from build123d import *

# Parameters (mm, degrees)
SKETCH1_W           = 63.5
SKETCH1_H           = 21.59
BOSS_EXTRUDE1_DEPTH = 5.08
SKETCH2_W           = 19.05
SKETCH2_H           = 20.32
BOSS_EXTRUDE2_DEPTH = 1.27
SKETCH3_W           = 1.27
SKETCH3_H           = 21.59
BOSS_EXTRUDE3_DEPTH = 20.32
SKETCH4_W           = 1.336000662
SKETCH4_H           = 43.13668157
BOSS_EXTRUDE4_DEPTH = 20.32
SKETCH5_W           = 10.16
SKETCH5_H           = 20.215193183
CUT_EXTRUDE2_DEPTH  = 1.27


with BuildPart() as part:
    # Sketch1 → Boss-Extrude1 (new body)
    with BuildSketch(Plane(origin=(0, 0, 0), x_dir=(1, 0, 0), z_dir=(0, 1, 0))):
        with Locations((-28.979219315, -15.643333637)):
            Rectangle(SKETCH1_W, SKETCH1_H)
    boss_extrude1 = extrude(amount=BOSS_EXTRUDE1_DEPTH)

    # Sketch2 → Boss-Extrude2 (add)
    with BuildSketch(Plane.XY.offset(26.438333637)):
        with Locations((-28.979219315, 15.24)):
            Rectangle(SKETCH2_W, SKETCH2_H)
    boss_extrude2 = extrude(amount=-BOSS_EXTRUDE2_DEPTH)

    # Sketch3 → Boss-Extrude3 (add)
    with BuildSketch(Plane(origin=(0, 5.08, 0), x_dir=(1, 0, 0), z_dir=(0, 1, 0))):
        with Locations((-39.139219315, -15.643333637)):
            Rectangle(SKETCH3_W, SKETCH3_H)
    boss_extrude3 = extrude(amount=BOSS_EXTRUDE3_DEPTH)

    # Mirror2: Boss-Extrude1, Boss-Extrude2, Boss-Extrude3 across plane
    add(boss_extrude1.mirror(Plane(origin=(-60.729219315, 5.08, 4.848333637), x_dir=(1, 0, 0), z_dir=(0, 0, 1))))
    add(boss_extrude2.mirror(Plane(origin=(-60.729219315, 5.08, 4.848333637), x_dir=(1, 0, 0), z_dir=(0, 0, 1))))
    add(boss_extrude3.mirror(Plane(origin=(-60.729219315, 5.08, 4.848333637), x_dir=(1, 0, 0), z_dir=(0, 0, 1))))

    # Sketch4 → Boss-Extrude4 (add)
    with BuildSketch(Plane(origin=(0, 5.08, 0), x_dir=(1, 0, 0), z_dir=(0, 1, 0))):
        with Locations((-18.786218984, -4.869992852)):
            Rectangle(SKETCH4_W, SKETCH4_H)
    extrude(amount=BOSS_EXTRUDE4_DEPTH)

    # Sketch5 → Cut-Extrude2 (cut)
    with BuildSketch(Plane(origin=(0, 0, -16.741666363), x_dir=(-1, 0, 0), z_dir=(0, 0, -1))):
        with Locations((29.613387645, 15.279515477)):
            Rectangle(SKETCH5_W, SKETCH5_H)
    extrude(amount=-CUT_EXTRUDE2_DEPTH, mode=Mode.SUBTRACT)


solid = part.part
Model file for the job. Use its own axes, mm. A direction names the side the tool comes from. Coordinates: 2 decimals unless noted, no trailing zeros. Write each loop counter-clockwise with the first axis right and the second up, starting at its lowest first coordinate (ties: lowest second). Pieces come first, ordered by that corner, then holes. Notation, with made-up numbers: (-36, 79) - (18, 79) arc R15 ccw to (18, 98) - close; hole circle Ø9 at (64, 86.25). An arc over 180 degrees is marked (long way). Write each question's results on one line, items separated by ' | '. Start each with the question number.
1) Cut at A-A (y = 21). Write the cut outline in (x, z).
2) Mould opens along Y. For faces 4 (the face through (-29, 4, -16.742)), 5 (the face through (-34.693, 15, -16)), 6 (the face through (-24.533, 15, -16)), 7 (the face through (-29, 5.08, 5)) say: pulls with the +Y half, pulls with the -Y half, needs draft (parallel to the pull), parting line crosses it, or undercut.
3) 3-axis set-ups, long thin cutter, end or side, ignore diameter. For faces 1 (the face through (-23, 15, -15.472)), 2 (the face through (-18.118, 15, 5)), 3 (the face through (-50, 5.08, 5)): which of +Z, -Z, +X, -X, +Y, -Y reach the whole face in a straight line?
4) Cut at C-C (z = -11). Write the cut outline in (x, y), then the cut area to 3 significant figures.
5) Cut at D-D (x = -54). Write the cut outline in (y, z).
6) Flat gauge pins, fed straight in: P1, Ø4, axis at x = -51.5, z = -3.5, coming from the +Y side; P2, Ø5.5, axis at x = -28.5, y = 13, coming from the -Z side; P3, Ø1, axis at y = 17, z = -16, coming from the -X side. Where does each tip first touch, or does it go through?
7) Cut at B-B (x = -21). Write the cut outline in (y, z).
8) Probe line 1 along X through (y, z) = (9.5, -2.5); line 2 along Y through (x, z) = (-50, -9.5). List the from-to ranges inside material, lowest first. Write a range as from..to.
Returned:
1) outline: (-39.77, -16.74) - (-34.69, -16.74) - (-34.69, -15.47) - (-38.5, -15.47) - (-38.5, 25.17) - (-19.45, 25.17) - (-19.45, -15.47) - (-24.53, -15.47) - (-24.53, -16.74) - (-19.45, -16.74) - (-19.45, -16.7) - (-18.12, -16.7) - (-18.12, 26.44) - (-39.77, 26.44) - close
2) face 4: needs draft | face 5: undercut | face 6: undercut | face 7: pulls with the +Y half
3) face 1: +Y | face 2: +Z, -Z, +X, +Y | face 3: +Z, -Z, -X, +Y
4) outline: (-60.73, 0) - (2.77, 0) - (2.77, 5.08) - (-18.12, 5.08) - (-18.12, 25.4) - (-19.45, 25.4) - (-19.45, 5.08) - (-38.5, 5.08) - (-38.5, 25.4) - (-39.77, 25.4) - (-39.77, 5.08) - (-60.73, 5.08) - close | area: 376 mm^2
5) outline: (0, -16.74) - (5.08, -16.74) - (5.08, 26.44) - (0, 26.44) - close
6) P1: y = 5.08 | P2: z = 25.17 | P3: x = -39.77
7) outline: (0, -16.74) - (25.4, -16.74) - (25.4, -15.47) - (5.08, -15.47) - (5.08, 25.17) - (25.4, 25.17) - (25.4, 26.44) - (0, 26.44) - close
8) line 1: -39.77..-38.5, -19.45..-18.12 | line 2: 0..5.08
